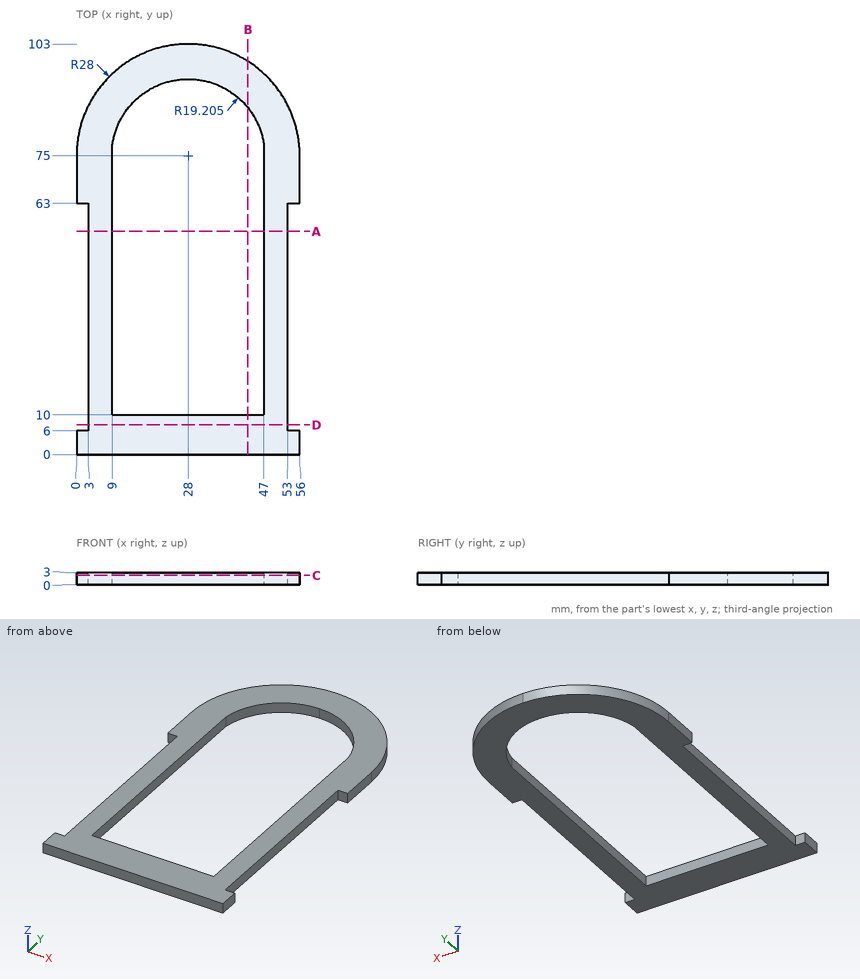
Answer from the drawing. Dimensions are ordinates in mm from the lowest x, y and z of the part. Round coordinates to 2 decimals unless told otherwise and drop trailing zeros. Loops run counter-clockwise (first coordinate to the right, second up) from the corner with the lowest first, then second, coordinate; pieces in that order, holes last. Notation, with made-up numbers: M 17,-26 L 54,-26 A20 ccw 54,9 Z; hole C -15.5,85.5 d4. An arc over 180 degrees is marked long. One line per question, with ' | ' between items. Start each with the question number.
(1) A cutting plane is placed at C-C on z = 2.35. Write down the section's boundary in (x, y) (1 decimal), plus the area to 3 significant figures.
(2) A cutting plane is placed at D-D on y = 7.5. Write down the section's boundary in (x, z).
(3) Flat-ended cylindrical pins translate along their axes: pin 1 Ø0.9 at (y, z) = (27, 1) entering from +X; pin 2 Ø1.5 at (x, z) = (27, 1) entering from +Y; pin 3 Ø1 at (x, z) = (13.5, 2) entering from +Y. Find the tip coordinate at first contact, or state that the pin passes through.
(4) Find the intervals of material crossed by line 1 (Y direction, x = 27.5, z = 1.75) (1 decimal); line 2 (X direction, y = 73.5, z = 1.5); line 3 (X direction, y = 61, z = 0.25), in increasing order.
(5) A cutting plane is placed at B-B on x = 43. Write down the section's boundary in (y, z).
(6) A cutting plane is placed at A-A on y = 56. Write down the section's boundary in (x, z).
Geometry check:
1) outline: M 0,0 L 56,0 L 56,6 L 53,6 L 53,63 L 56,63 L 56,75 A28 ccw 0,75 L 0,63 L 3,63 L 3,6 L 0,6 Z; hole M 9,10 L 47,10 L 47,77.8 A19.2 ccw 9,77.8 Z | area: 2,040 mm²
2) outline: M 3,0 L 53,0 L 53,3 L 3,3 Z
3) pin 1: stops at x = 53 | pin 2: stops at y = 103 | pin 3: stops at y = 99.25
4) line 1: y = 0 to 10, 94.2 to 103 | line 2: x = 0 to 9, 47 to 56 | line 3: x = 3 to 9, 47 to 53
5) outline: M 0,0 L 10,0 L 10,3 L 0,3 Z; M 86.99,0 L 98.64,0 L 98.64,3 L 86.99,3 Z
6) outline: M 3,0 L 9,0 L 9,3 L 3,3 Z; M 47,0 L 53,0 L 53,3 L 47,3 Z
